Print and shaded views of the part. All mm, measured from the part's lowest x, y and z. Coordinates: 2 decimals unless noted, no trailing zeros. Order: outer loops, then holes, each group sorted by start corner. A loop starts at its lowest first (then second) coordinate and runs counter-clockwise, first axis right, second up. Notation, with made-up numbers: M 83.25,19 L 132.25,19 A30 ccw 132.25,47 Z; hole C -6,53 d6. An arc over 180 degrees is marked long. One line per item, written item: value.
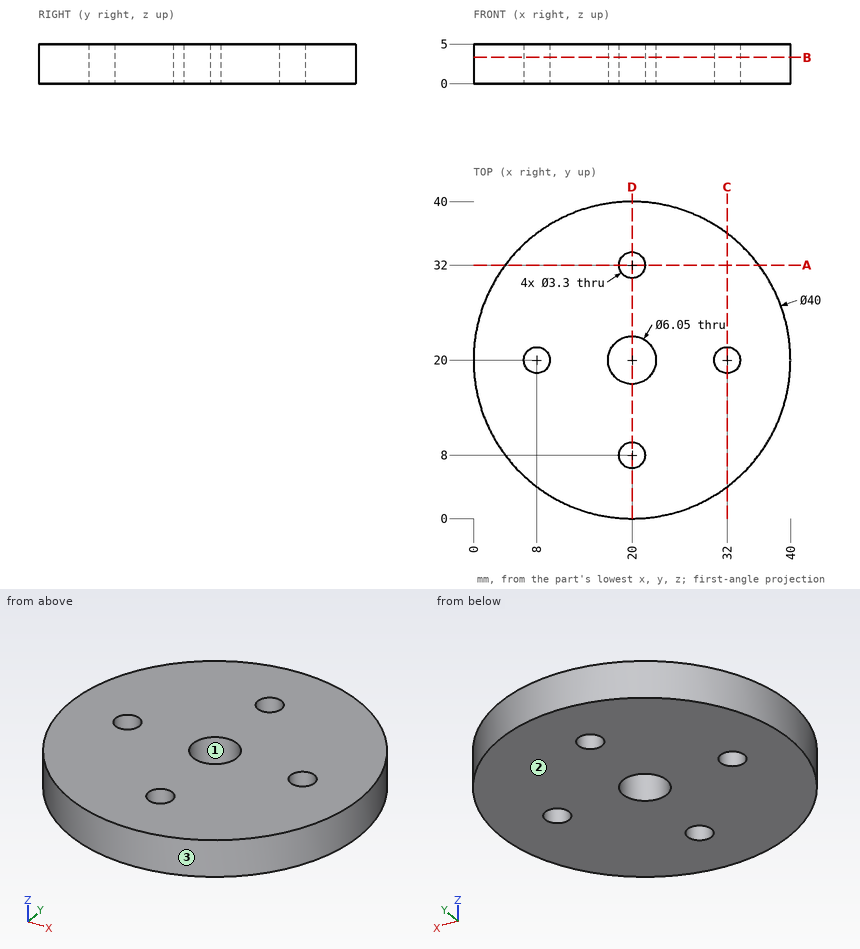
Q1. Slice it at B-B (z = 3.3). List the corners of the cut face in (x, y) (3 decimals).
Recorded:
outline: C 20,20 d40; hole C 8,20 d3.3; hole C 20,20 d6.05; hole C 20,8 d3.3; hole C 20,32 d3.3; hole C 32,20 d3.3
Q2. Slice it at D-D (x = 20). List the corners of the cut face in (y, z) (3 decimals).
Recorded:
outline: M 0,0 L 6.35,0 L 6.35,5 L 0,5 Z; M 9.65,0 L 16.975,0 L 16.975,5 L 9.65,5 Z; M 23.025,0 L 30.35,0 L 30.35,5 L 23.025,5 Z; M 33.65,0 L 40,0 L 40,5 L 33.65,5 Z
Q3. Drill centre lines: line 1 along Y through (x, z) = (20, 3.6) (3 decimals); line 2 along Y through (x, z) = (18.5, 1.95); line 3 along X through (y, z) = (18, 1.45). Where is each one in solid material? Low to high.
Recorded:
line 1: y = 0 to 6.35, 9.65 to 16.975, 23.025 to 30.35, 33.65 to 40
line 2: y = 0.06 to 7.31, 8.69 to 17.37, 22.63 to 31.31, 32.69 to 39.94
line 3: x = 0.1 to 17.73, 22.27 to 39.9
Q4. Slice it at A-A (y = 32). List the corners of the cut face in (x, z), plus the area to 4 significant figures.
Recorded:
outline: M 4,0 L 18.35,0 L 18.35,5 L 4,5 Z; M 21.65,0 L 36,0 L 36,5 L 21.65,5 Z
area: 143.5 mm^2
Q5. Mould opens along X. For the marked faces 1, 2 and 3 say: released by +X, released by -X, zero draft, split by the parting line, or undercut.
Recorded:
face 1: undercut
face 2: zero draft
face 3: split by the parting line
Q6. Pin check, flat tips, straight feed: pin 1 Ø2 at (y, z) = (13, 3.5) entering from +X; pin 2 Ø2 at (x, z) = (25.5, 0.5) entering from -Y; pin 3 Ø3 at (y, z) = (32.5, 1) entering from +X. Stop position of each tip, or through.
Recorded:
pin 1: stops at x = 39.08
pin 2: stops at y = 0.51
pin 3: stops at x = 36.7
